Work out the finished part from the listing and answer in its coordinate system (mm). A direction names the side the tool comes from. Round coordinates to 2 decimals unless told otherwise and drop trailing zeros. Write each loop counter-clockwise with the first axis right and the second up, starting at its lowest first coordinate (ties: lowest second). Pieces come first, ordered by that corner, then holes. Notation, with made-up numbers: M -17,73 L -10,73 A16 cw -10,88 Z; hole C -3.5,-37 d8. An arc over 180 degrees is marked long. Answer in a Markdown table with one row per item.
```python
from build123d import *

# Parameters (mm, degrees)
SKETCH1_R           = 0.840105
SKETCH1_R_2         = 1.190625
BOSS_EXTRUDE1_DEPTH = 3.175


with BuildPart() as part:
    # Sketch1 → Boss-Extrude1 (new body)
    with BuildSketch(Plane(origin=(0, 0, 0), x_dir=(1, 0, 0), z_dir=(0, 1, 0))):
        with BuildLine():
            Line((-13.027020503, 16.390799837), (-13.027020503, 36.710799837))
            ThreePointArc((-13.027020503, 36.710799837), (-10.379674956, 39.495223926), (-6.677020503, 40.520799837))
            ThreePointArc((-6.677020503, 40.520799837), (-2.974366049, 39.495223926), (-0.327020503, 36.710799837))
            Line((-0.327020503, 36.710799837), (-0.327020503, 16.390799837))
            Line((-0.327020503, 16.390799837), (13.277400654, 3.055799837))
            Line((13.277400654, 3.055799837), (13.277400654, -3.294200163))
            ThreePointArc((13.277400654, -3.294200163), (9.685298205, -4.782097715), (8.197400654, -8.374200163))
            Line((8.197400654, -8.374200163), (8.197400654, -47.744200163))
            ThreePointArc((8.197400654, -47.744200163), (9.685298205, -51.336302612), (13.277400654, -52.824200163))
            Line((13.277400654, -52.824200163), (13.277400654, -60.444200163))
            ThreePointArc((13.277400654, -60.444200163), (4.297144533, -56.724456284), (0.577400654, -47.744200163))
            Line((0.577400654, -47.744200163), (0.577400654, 3.055799837))
            Line((0.577400654, 3.055799837), (-13.027020503, 16.390799837))
        make_face()
        with Locations((-6.677020503, 27.820799837)):
            Circle(SKETCH1_R, mode=Mode.SUBTRACT)
        with Locations((-6.677020503, 36.710799837)):
            Circle(SKETCH1_R_2, mode=Mode.SUBTRACT)
        with BuildLine():
            Line((-2.63294069, 14.03829086), (4.529585854, 7.097736719))
            ThreePointArc((4.529585854, 7.097736719), (4.551571997, 5.389416502), (2.843251781, 5.367430359))
            Line((2.843251781, 5.367430359), (-4.24408648, 12.394593219))
            ThreePointArc((-4.24408648, 12.394593219), (-4.260362405, 14.022014935), (-2.63294069, 14.03829086))
        make_face(mode=Mode.SUBTRACT)
    extrude(amount=BOSS_EXTRUDE1_DEPTH)


solid = part.part
```
1. The part is cut by section D-D (x = 11.75). Determine the outline of the cut face in (y, z) (3 decimals).
Calculated:
| item | result |
|---|---|
| outline | M 0,-4.553 L 3.175,-4.553 L 3.175,3.529 L 0,3.529 Z; M 0,52.589 L 3.175,52.589 L 3.175,60.352 L 0,60.352 Z |
2. Determine the mould class of faces 1 (the flat face through (-6.1, 1.6, -9.6)), 2 (the flat face through (6.38, 1.565, -9.817)), 3 (the flat face through (-0.327, 2, -27)), 4 (the flat face through (-0.65, 1.57, -8.83)) for opening direction Z: released by +Z, released by -Z, zero draft, split by the parting line, or undercut.
Calculated:
| item | result |
|---|---|
| face 1 | released by +Z |
| face 2 | released by -Z |
| face 3 | zero draft |
| face 4 | undercut |
3. The part is cut by section B-B (y = 2.25). Determine the outline of the cut face in (x, z), plus the area to 3 significant figures.
Calculated:
| item | result |
|---|---|
| outline | M -13.03,-36.71 A7.2 ccw -0.33,-36.71 L -0.33,-16.39 L 13.28,-3.06 L 13.28,3.29 A5.08 cw 8.2,8.37 L 8.2,47.74 A5.08 cw 13.28,52.82 L 13.28,60.44 A12.7 ccw 0.58,47.74 L 0.58,-3.06 L -13.03,-16.39 Z; hole C -6.68,-36.71 d2.38; hole C -6.68,-27.82 d1.68; hole M -4.24,-12.39 A1.15 ccw -2.63,-14.04 L 4.53,-7.1 A1.21 ccw 2.84,-5.37 Z |
| area | 959 mm² |
4. The part is cut by section C-C (z = -26). Determine the outline of the cut face in (x, y) (3 decimals).
Calculated:
| item | result |
|---|---|
| outline | M -13.027,0 L -0.327,0 L -0.327,3.175 L -13.027,3.175 Z |
5. The part is cut by section A-A (x = -1.25). Determine the outline of the cut face in (y, z) (3 decimals), plus the area to 3 significant figures.
Calculated:
| item | result |
|---|---|
| outline | M 0,-38.051 L 3.175,-38.051 L 3.175,-12.698 L 0,-12.698 Z; M 0,-9.426 L 3.175,-9.426 L 3.175,-4.847 L 0,-4.847 Z |
| area | 95.0 mm² |
6. Given pin 1 (12 mm diameter, centred on x = -3, z = 26.5, fed in from -Y); pin 2 (1.6 mm diameter, centred on y = 1, z = -21.5, fed in from +X); pin 3 (1 mm diameter, centred on x = 8, y = 1, fed in from -Z); pin 4 (1 mm diameter, centred on y = 1, z = 25, fed in from -X), each flat-ended and moving along its own axis, determine where each tip first touches the part or whether it passes through.
Calculated:
| item | result |
|---|---|
| pin 1 | stops at y = 0 |
| pin 2 | stops at x = -0.33 |
| pin 3 | stops at z = -8.72 |
| pin 4 | stops at x = 0.58 |
7. A tool of negligible diameter and unlimited length cuts with its end or side. For faces 5 (the flat face through (0.898, 1.565, -10.617)), 6 (the flat face through (0.577, 2, 23)), 7 (the cylindrical face through (9.73, 1.57, 4.74)), from which of +Z, -Z, +X, -X, +Y, -Y can it reach the whole face along a straight path? Write none if from no direction.
Calculated:
| item | result |
|---|---|
| face 5 | +Y, -Y |
| face 6 | +Z, -X, +Y, -Y |
| face 7 | +X, +Y, -Y |
8. Consider line 1 along Z through (x, y) = (-3.75, 1.3); line 2 along Z through (x, y) = (-6.75, 2.8); line 3 along Z through (x, y) = (9.75, 1.75). Determine where each line is inside the solid, lowest interval first. Write a range as from..to.
Calculated:
| item | result |
|---|---|
| line 1 | z = -39.9..-14.32, -11.9..-7.3 |
| line 2 | z = -40.52..-37.9, -35.52..-28.66, -26.98..-10.24 |
| line 3 | z = -6.51..4.72, 51.4..59.94 |
